Geometry: final body of the model. Coordinates: model frame, mm. A direction names the side the tool comes from. Coordinates: 2 decimals unless noted, no trailing zeros. Write each loop counter-clockwise with the first axis right and the second up, starting at its lowest first coordinate (ties: lowest second). Pieces come first, ordered by that corner, then holes. Notation, with made-up numbers: (72, 78.25) -> (99, 78.25) arc R28 ccw to (99, 114.25) -> close; hole circle Ø3 at (-11, 30). An arc over 180 degrees is marked (long way). Answer as a JSON object with one key per item and string values. Group by question number.
```python
from build123d import *

# Parameters (mm, degrees)
SALIENTE_EXTRUIR1_DEPTH = 15
CROQUIS4_W              = 2
CROQUIS4_H              = 6
SALIENTE_EXTRUIR2_DEPTH = 15
CROQUIS5_R              = 2.575
CORTAR_EXTRUIR1_DEPTH   = 4
CROQUIS6_W              = 17.65
CROQUIS6_H              = 5
SALIENTE_EXTRUIR3_DEPTH = 15
CROQUIS7_R              = 2.825
CORTAR_EXTRUIR2_DEPTH   = 5
CROQUIS8_R              = 1.75
CORTAR_EXTRUIR3_DEPTH   = 13.8


with BuildPart() as part:
    # Croquis2 → Saliente-Extruir1 (new body)
    with BuildSketch(Plane(origin=(0, 0, 0), x_dir=(0, 0, -1), z_dir=(1, 0, 0))):
        Polygon((0, 0), (13, 0), (13, 9.8), (25.65, 9.8), (25.65, 12.8), (10, 12.8), (10, 3), (0, 3), align=None)
    extrude(amount=SALIENTE_EXTRUIR1_DEPTH)

    # Croquis4 → Saliente-Extruir2 (add, through all)
    with BuildSketch(Plane(origin=(0, 0, 0), x_dir=(0, 0, -1), z_dir=(1, 0, 0))):
        with Locations((26.65, 9.8)):
            Rectangle(CROQUIS4_W, CROQUIS4_H)
    extrude(amount=SALIENTE_EXTRUIR2_DEPTH)

    # Croquis5 → Cortar-Extruir1 (cut, through all)
    with BuildSketch(Plane(origin=(0, 3, 0), x_dir=(1, 0, 0), z_dir=(0, 1, 0))):
        with Locations((7.5, 5)):
            Circle(CROQUIS5_R)
    extrude(amount=-CORTAR_EXTRUIR1_DEPTH, mode=Mode.SUBTRACT)

    # Croquis6 → Saliente-Extruir3 (add)
    with BuildSketch(Plane(origin=(15, 0, 0), x_dir=(0, 0, -1), z_dir=(1, 0, 0))):
        with Locations((18.825, 15.3)):
            Rectangle(CROQUIS6_W, CROQUIS6_H)
    extrude(amount=-SALIENTE_EXTRUIR3_DEPTH)

    # Croquis7 → Cortar-Extruir2 (cut)
    with BuildSketch(Plane(origin=(0, 17.8, 0), x_dir=(1, 0, 0), z_dir=(0, 1, 0))):
        with Locations((7.5, 18.825)):
            Circle(CROQUIS7_R)
    extrude(amount=-CORTAR_EXTRUIR2_DEPTH, mode=Mode.SUBTRACT)

    # Croquis8 → Cortar-Extruir3 (cut, through all)
    with BuildSketch(Plane(origin=(0, 12.8, 0), x_dir=(1, 0, 0), z_dir=(0, 1, 0))):
        with Locations((7.5, 18.825)):
            Circle(CROQUIS8_R)
    extrude(amount=-CORTAR_EXTRUIR3_DEPTH, mode=Mode.SUBTRACT)


solid = part.part
```
Item 1: Mould query, pull axis X, two halves, no side actions, for faces 1 (the cylindrical face through (10.195, 15.335, -19.674)), 2 (the flat face through (7, 5, -13)), 3 (the flat face through (15, 11, -17)). Classes: +X half, -X half, draft (parallel to the pull), parting line (faces both ways), or undercut.
Item 2: Contact query for flat-ended pins moving along their axis: pin 1 (3 mm diameter, centred on x = 2.5, z = -8.5, fed in from -Y); pin 2 (2 mm diameter, centred on x = 11.5, z = -6, fed in from +Y); pin 3 (1.6 mm diameter, centred on x = 9, z = -26.5, fed in from -Y); pin 4 (1 mm diameter, centred on x = 5.5, y = 7.5, fed in from +Z). Output: stop coordinate, or through.
Item 3: Ray query, L1, parallel to Z at x = 1.75, y = 7.75; L2, parallel to Z at x = 7.5, y = 11.5 (3 decimals); L3, parallel to X at y = 2.15, z = -5 (3 decimals). Return the intervals inside material, ascending. Write a range as [from, to].
Item 4: Section D-D on z = -22.25. Output: boundary loops of the cut face in (x, y).
Item 5: Section A-A on x = 7.5. Output: boundary loops of the cut face in (y, z) (3 decimals).
Item 6: Section B-B on x = 12.5. Output: boundary loops of the cut face in (y, z), then the cut area to 3 significant figures.
Item 7: Set-up query: faces 4 (the flat face through (5.7, 3, -2.8)), 5 (the flat face through (7, 9.8, -21)), 6 (the flat face through (9, 12.8, -20)). Return all of +Z, -Z, +X, -X, +Y, -Y with unobstructed straight access to the full face (end or side cutting, diameter ignored); none if empty.
Item 8: Section C-C on y = 10.5. Output: boundary loops of the cut face in (x, z) (3 decimals), then the cut area to 3 significant figures.
Answer sheet:
{
 "1": {"face 1": "undercut", "face 2": "draft", "face 3": "+X half"},
 "2": {"pin 1": "stops at y = 0", "pin 2": "stops at y = 3", "pin 3": "stops at y = 6.8", "pin 4": "stops at z = -10"},
 "3": {"L1": "z = [-27.65, -25.65], [-13, -10]", "L2": "z = [-27.65, -20.575], [-17.075, -10]", "L3": "x = [0, 4.925], [10.075, 15]"},
 "4": {"outline": "(0, 9.8) -> (15, 9.8) -> (15, 17.8) -> (0, 17.8) -> close"},
 "5": {"outline": "(0, -13) -> (9.8, -13) -> (9.8, -17.075) -> (12.8, -17.075) -> (12.8, -16) -> (17.8, -16) -> (17.8, -10) -> (3, -10) -> (3, -7.575) -> (0, -7.575) -> close; (0, -2.425) -> (3, -2.425) -> (3, 0) -> (0, 0) -> close; (6.8, -27.65) -> (17.8, -27.65) -> (17.8, -21.65) -> (12.8, -21.65) -> (12.8, -20.575) -> (9.8, -20.575) -> (9.8, -25.65) -> (6.8, -25.65) -> close"},
 "6": {"outline": "(0, -13) -> (9.8, -13) -> (9.8, -25.65) -> (6.8, -25.65) -> (6.8, -27.65) -> (17.8, -27.65) -> (17.8, -10) -> (3, -10) -> (3, 0) -> (0, 0) -> close", "area": "207 mm^2"},
 "7": {"face 4": "+Z, +X, -X, +Y", "face 5": "+X, -X, -Y", "face 6": "+Y"},
 "8": {"outline": "(0, -27.65) -> (15, -27.65) -> (15, -10) -> (0, -10) -> close; hole circle Ø3.5 at (7.5, -18.825)", "area": "255 mm^2"}
}
